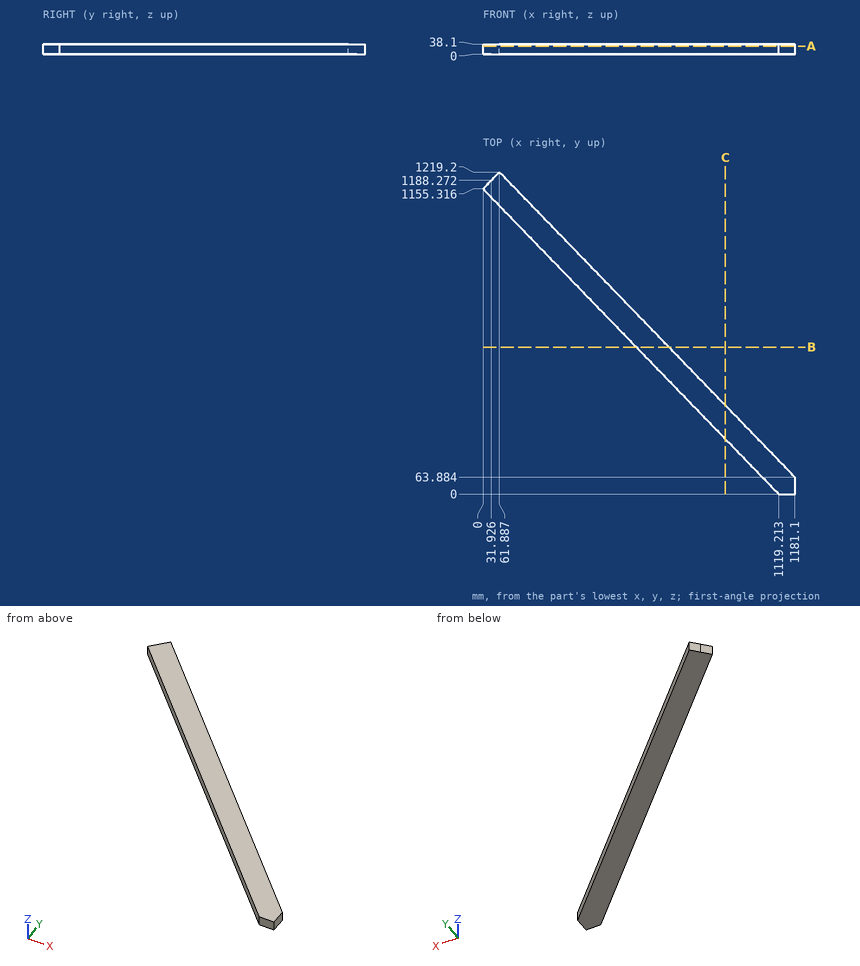
Could you check a few things on this drawing? It's one solid part, dimensions in mm from its lowest x, y, z. Round coordinates to 2 decimals unless told otherwise and drop trailing zeros. Order: outer loops, then holes, each group sorted by start corner. A loop starts at its lowest first (then second) coordinate and runs counter-clockwise, first axis right, second up.
(1) Imagine slicing it at A-A (z = 30.5). Write out the boundary of the cut face in (x, y) (1 decimal), plus the area to 3 significant figures.
Response values:
outline: (0, 1155.3) - (1119.2, 0) - (1181.1, 0) - (1181.1, 63.9) - (61.9, 1219.2) - close
area: 145,000 mm2
(2) Imagine slicing it at B-B (y = 556). Write out the boundary of the cut face in (x, z).
Response values:
outline: (580.59, 0) - (704.36, 0) - (704.36, 38.1) - (580.59, 38.1) - close
(3) I'm going to push flat-ended pins straight in: pin 1 (10 mm diameter, centred on x = 572.5, z = 14.5, fed in from +Y); pin 2 (2 mm diameter, centred on x = 270, z = 16.5, fed in from -Y) (1 decimal); pin 3 (1 mm diameter, centred on y = 818.5, z = 21, fed in from +X). Where does each tip first touch, or does it pass through?
Response values:
pin 1: stops at y = 697.28
pin 2: stops at y = 875.6
pin 3: stops at x = 450.55
(4) Please list where these lines run through material, in increasing order: line 1 along Y through (x, z) = (1065, 33); line 2 along X through (y, z) = (65, 6) (1 decimal); line 3 along X through (y, z) = (563, 29) (1 decimal).
Response values:
line 1: y = 55.96 to 183.73
line 2: x = 1056.2 to 1180
line 3: x = 573.8 to 697.6
(5) Imagine slicing it at C-C (x = 917.5). Write out the boundary of the cut face in (y, z), plus the area to 3 significant figures.
Response values:
outline: (208.22, 0) - (335.99, 0) - (335.99, 38.1) - (208.22, 38.1) - close
area: 4,870 mm2
